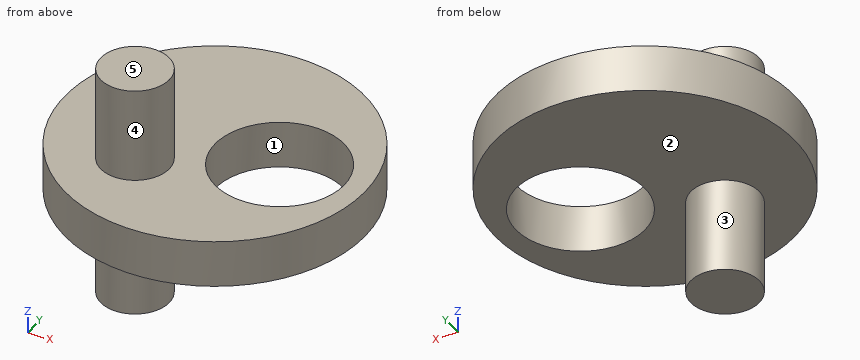
from build123d import *

# Parameters (mm, degrees)
F0_R          = 31.728822
F0_R_2        = 13.666047
F1_DEPTH      = 5
F1_DEPTH_BACK = 5
F2_R          = 7.26181
F3_DEPTH      = 25
F3_DEPTH_BACK = 25


with BuildPart() as f1:
    # F0 (on Top) → F1 (new body, two sides)
    with BuildSketch(Plane.XY) as f1_sk:
        Circle(F0_R)
        with Locations((13.666047, 0)):
            Circle(F0_R_2, mode=Mode.SUBTRACT)
    extrude(amount=F1_DEPTH)
    extrude(f1_sk.sketch, amount=-F1_DEPTH_BACK)

    # F2 (on Top) → F3 (join, two sides)
    with BuildSketch(Plane.XY) as f3_sk:
        with Locations((-10.615021, -11.218742)):
            Circle(F2_R)
    extrude(amount=F3_DEPTH)
    extrude(f3_sk.sketch, amount=-F3_DEPTH_BACK)


solid = f1.part
The listing builds one solid part. Answer for the finished solid, in the listing's coordinates (mm). Face numbers are marked on the shaded views. A direction names the side the tool comes from. Give positions to 0.01 mm unless a question says otherwise; leave off trailing zeros. Loops run counter-clockwise (first coordinate to the right, second up) from the corner with the lowest first, then second, coordinate; pieces in that order, holes last.
Item 1: Determine the mould class of the marked faces 1, 2 and 3 for opening direction X: +X half, -X half, draft (parallel to the pull), parting line (faces both ways), or undercut.
Derived:
face 1: undercut
face 2: draft
face 3: parting line
Item 2: A tool of negligible diameter and unlimited length cuts with its end or side. For the marked faces 4 and 5, from which of +Z, -Z, +X, -X, +Y, -Y can it reach the whole face along a straight path? Write none if from no direction.
Derived:
face 4: +Z
face 5: +Z, +X, -X, +Y, -Y
Item 3: A cutting plane is placed at D-D (y = -17.5). Give the vertices of the cut face in (x, z), then the cut area to 3 significant figures.
Derived:
outline: (-26.47, -5) - (-14.26, -5) - (-14.26, -25) - (-6.97, -25) - (-6.97, -5) - (26.47, -5) - (26.47, 5) - (-6.97, 5) - (-6.97, 25) - (-14.26, 25) - (-14.26, 5) - (-26.47, 5) - close
area: 821 mm2
Item 4: A cutting plane is placed at C-C (z = -2.5). Give the vertices of the cut face in (x, y).
Derived:
outline: circle Ø63.46 at (0, 0); hole circle Ø27.33 at (13.67, 0)
Item 5: Find the intervals of material crossed by line 1 along Z through (x, y) = (-21, 17); line 2 along Y through (x, z) = (12, -3.5); line 3 along Y through (x, z) = (17, -2), in increasing order.
Derived:
line 1: z = -5 to 5
line 2: y = -29.37 to -13.56, 13.56 to 29.37
line 3: y = -26.79 to -13.25, 13.25 to 26.79
Item 6: A cutting plane is placed at B-B (x = 1). Give the vertices of the cut face in (y, z), then the cut area to 3 significant figures.
Derived:
outline: (-31.71, -5) - (-5.13, -5) - (-5.13, 5) - (-31.71, 5) - close; (5.13, -5) - (31.71, -5) - (31.71, 5) - (5.13, 5) - close
area: 532 mm2
Item 7: Each of these flat-tipped pins is pushed along its axis until it touches: pin 1 Ø2 at (x, z) = (-21, 5.5) entering from -Y; pin 2 Ø19 at (x, y) = (-1.5, 5) entering from -Z; pin 3 Ø4 at (x, z) = (-14, -3) entering from +Y. Where does it stop, or does it pass through?
Derived:
pin 1: stops at y = -24.52
pin 2: stops at z = -5
pin 3: stops at y = 29.37
Item 8: A cutting plane is placed at A-A (y = 0). Give the vertices of the cut face in (x, z), then the cut area to 3 significant figures.
Derived:
outline: (-31.73, -5) - (0, -5) - (0, 5) - (-31.73, 5) - close; (27.33, -5) - (31.73, -5) - (31.73, 5) - (27.33, 5) - close
area: 361 mm2
